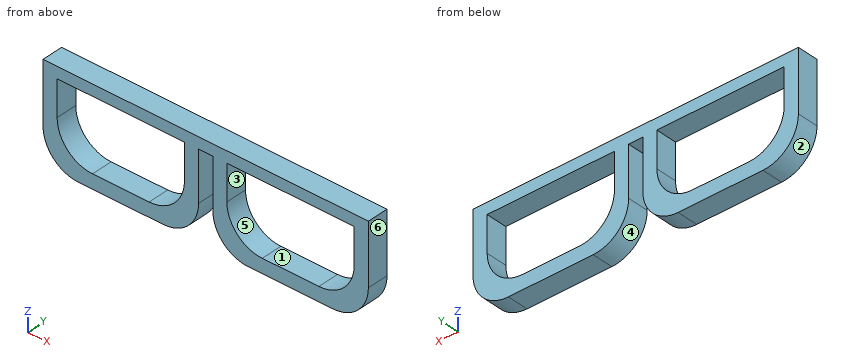
from build123d import *

# Parameters (mm, degrees)
F0_W     = 2.54
F0_H     = 2.2360555756
F1_DEPTH = 1.905


with BuildPart() as f1:
    # F0 (on Front) → F1 (new body, symmetric)
    with BuildSketch(Plane.XZ):
        Polygon((-58.3446317705, 24.4664963263), (-55.8046317705, 24.4664963263), (-32.9446317705, 24.4664963263), (-30.4046317705, 24.4664963263), (-27.8646317705, 24.4664963263), (-25.3246317705, 24.4664963263), (-2.4646317705, 24.4664963263), (0.0753682295, 24.4664963263), (0.0753682295, 26.4984963263), (-58.3446317705, 26.4984963263), align=None)
        with BuildLine():
            Line((-55.8046317705, 18.1164963263), (-55.8046317705, 24.4664963263))
            Line((-55.8046317705, 24.4664963263), (-58.3446317705, 24.4664963263))
            Line((-58.3446317705, 24.4664963263), (-58.3446317705, 15.5880270362))
            ThreePointArc((-58.3446317705, 15.5880270362), (-56.484759831, 11.0978989757), (-51.9946317705, 9.2380270362))
            Line((-51.9946317705, 9.2380270362), (-36.7546317705, 9.2380270362))
            ThreePointArc((-36.7546317705, 9.2380270362), (-32.2645037099, 11.0978989757), (-30.4046317705, 15.5880270362))
            Line((-30.4046317705, 15.5880270362), (-30.4046317705, 22.2304407507))
            Line((-30.4046317705, 22.2304407507), (-32.9446317705, 22.2304407507))
            Line((-32.9446317705, 22.2304407507), (-32.9446317705, 18.1164963263))
            ThreePointArc((-32.9446317705, 18.1164963263), (-34.8045037099, 13.6263682658), (-39.2946317705, 11.7664963263))
            Line((-39.2946317705, 11.7664963263), (-49.4546317705, 11.7664963263))
            ThreePointArc((-49.4546317705, 11.7664963263), (-53.944759831, 13.6263682658), (-55.8046317705, 18.1164963263))
        make_face()
        with BuildLine():
            Line((-25.3246317705, 22.2304407507), (-27.8646317705, 22.2304407507))
            Line((-27.8646317705, 22.2304407507), (-27.8646317705, 15.5880270362))
            ThreePointArc((-27.8646317705, 15.5880270362), (-26.004759831, 11.0978989757), (-21.5146317705, 9.2380270362))
            Line((-21.5146317705, 9.2380270362), (-6.2746317705, 9.2380270362))
            ThreePointArc((-6.2746317705, 9.2380270362), (-1.7845037099, 11.0978989757), (0.0753682295, 15.5880270362))
            Line((0.0753682295, 15.5880270362), (0.0753682295, 24.4664963263))
            Line((0.0753682295, 24.4664963263), (-2.4646317705, 24.4664963263))
            Line((-2.4646317705, 24.4664963263), (-2.4646317705, 18.1164963263))
            ThreePointArc((-2.4646317705, 18.1164963263), (-4.3245037099, 13.6263682658), (-8.8146317705, 11.7664963263))
            Line((-8.8146317705, 11.7664963263), (-18.9746317705, 11.7664963263))
            ThreePointArc((-18.9746317705, 11.7664963263), (-23.464759831, 13.6263682658), (-25.3246317705, 18.1164963263))
            Line((-25.3246317705, 18.1164963263), (-25.3246317705, 22.2304407507))
        make_face()
        with Locations((-26.5946317705, 23.3484685385)):
            Rectangle(F0_W, F0_H)
        with Locations((-31.6746317705, 23.3484685385)):
            Rectangle(F0_W, F0_H)
    extrude(amount=F1_DEPTH, both=True)


solid = f1.part
Check sheet for the modelled part. Datum: model origin and axes. Units: mm. Face numbers are marked on the shaded views. A direction names the side the tool comes from. Coordinates: 2 decimals unless noted, no trailing zeros. Write each loop counter-clockwise with the first axis right and the second up, starting at its lowest first coordinate (ties: lowest second). Pieces come first, ordered by that corner, then holes.
Item 1: Cross-section at A-A on z = 22. Record the boundary of the cut face in (x, y) (3 decimals), then the cut area to 3 significant figures.
Numbers:
outline: (-58.345, -1.905) - (-55.805, -1.905) - (-55.805, 1.905) - (-58.345, 1.905) - close; (-32.945, -1.905) - (-30.405, -1.905) - (-30.405, 1.905) - (-32.945, 1.905) - close; (-27.865, -1.905) - (-25.325, -1.905) - (-25.325, 1.905) - (-27.865, 1.905) - close; (-2.465, -1.905) - (0.075, -1.905) - (0.075, 1.905) - (-2.465, 1.905) - close
area: 38.7 mm2
Item 2: Cross-section at B-B on y = 0.9. Record the boundary of the cut face in (x, z).
Numbers:
outline: (-58.34, 15.59) arc R6.35 ccw to (-51.99, 9.24) - (-36.75, 9.24) arc R6.35 ccw to (-30.4, 15.59) - (-30.4, 24.47) - (-27.86, 24.47) - (-27.86, 15.59) arc R6.35 ccw to (-21.51, 9.24) - (-6.27, 9.24) arc R6.35 ccw to (0.08, 15.59) - (0.08, 26.5) - (-58.34, 26.5) - close; hole (-55.8, 18.12) arc R6.35 ccw to (-49.45, 11.77) - (-39.29, 11.77) arc R6.35 ccw to (-32.94, 18.12) - (-32.94, 24.47) - (-55.8, 24.47) - close; hole (-25.32, 18.12) arc R6.35 ccw to (-18.97, 11.77) - (-8.81, 11.77) arc R6.35 ccw to (-2.46, 18.12) - (-2.46, 24.47) - (-25.32, 24.47) - close
Item 3: Depth check by flat-ended pin: pin 1 Ø1.3 at (x, y) = (-29, 0.5) entering from -Z; pin 2 Ø3 at (x, z) = (-16.5, 13.5) entering from +Y. Enter the tip coordinate at first touch or a pass-through.
Numbers:
pin 1: stops at z = 24.47
pin 2: passes through
Item 4: Mould release check, pull along Z, two halves, no side actions. Record for the marked faces 3, 4, 5 and 6: released by +Z, released by -Z, zero draft, split by the parting line, or undercut.
Numbers:
face 3: undercut
face 4: released by -Z
face 5: undercut
face 6: zero draft
Item 5: Access from +Z, -Z, +X, -X, +Y, -Y to the whole of each face (thin tool, end or side, straight path). Record for the marked faces 1 and 2.
Numbers:
face 1: +Y, -Y
face 2: -Z, -X, +Y, -Y
Item 6: Cross-section at C-C on x = -7.5. Record the boundary of the cut face in (y, z) (1 decimal).
Numbers:
outline: (-1.9, 9.2) - (1.9, 9.2) - (1.9, 11.9) - (-1.9, 11.9) - close; (-1.9, 24.5) - (1.9, 24.5) - (1.9, 26.5) - (-1.9, 26.5) - close
Item 7: Cross-section at D-D on x = -43. Record the boundary of the cut face in (y, z) (1 decimal), then the cut area to 3 significant figures.
Numbers:
outline: (-1.9, 9.2) - (1.9, 9.2) - (1.9, 11.8) - (-1.9, 11.8) - close; (-1.9, 24.5) - (1.9, 24.5) - (1.9, 26.5) - (-1.9, 26.5) - close
area: 17.4 mm2
Item 8: Scan lines: probe 1 along X at (y, z) = (-0.95, 23.25); probe 2 along X at (y, z) = (0.7, 17.75); probe 3 along Z at (x, y) = (-13, -1.55). Record each from-to range of solid material in increasing order.
Numbers:
probe 1: x = -58.34 to -55.8, -32.94 to -30.4, -27.86 to -25.32, -2.46 to 0.08
probe 2: x = -58.34 to -55.79, -32.96 to -30.4, -27.86 to -25.31, -2.48 to 0.08
probe 3: z = 9.24 to 11.77, 24.47 to 26.5
